```python
from build123d import *

# Parameters (mm, degrees)
BOSS_EXTRUDE1_START     = -5
BOSS_EXTRUDE1_OUTLINE_W = 200
BOSS_EXTRUDE1_OUTLINE_H = 70
BOSS_EXTRUDE1_OUTLINE_R = 2.25
BOSS_EXTRUDE1_DEPTH     = 5
BOSS_EXTRUDE2_START     = 3
SKETCH2_W               = 200
SKETCH2_H               = 65
SKETCH2_R               = 2.25
BOSS_EXTRUDE2_DEPTH     = 3
CHAMFER1_SIZE           = 8
CHAMFER3_SIZE           = 3
SKETCH3_W               = 7.071067812
SKETCH3_H               = 2.6
CUT_EXTRUDE1_DEPTH      = 224.573349607


# Read off the part's stored shape, not the designer's step: Boss-Extrude1
with BuildPart() as part:
    # Boss-Extrude1 outline → Boss-Extrude1 (new body)
    with BuildSketch(Plane.XY.offset(BOSS_EXTRUDE1_START)):
        with Locations((100, 35)):
            Rectangle(BOSS_EXTRUDE1_OUTLINE_W, BOSS_EXTRUDE1_OUTLINE_H)
        with Locations((20, 9)):
            Circle(BOSS_EXTRUDE1_OUTLINE_R, mode=Mode.SUBTRACT)
        with Locations((180, 9)):
            Circle(BOSS_EXTRUDE1_OUTLINE_R, mode=Mode.SUBTRACT)
        with Locations((20, 58)):
            Circle(BOSS_EXTRUDE1_OUTLINE_R, mode=Mode.SUBTRACT)
        with Locations((180, 58)):
            Circle(BOSS_EXTRUDE1_OUTLINE_R, mode=Mode.SUBTRACT)
    extrude(amount=BOSS_EXTRUDE1_DEPTH)

    # Sketch2 → Boss-Extrude2 (add)
    with BuildSketch(Plane(origin=(0, 0, -5), x_dir=(-1, 0, 0), z_dir=(0, 0, -1)).offset(BOSS_EXTRUDE2_START)):
        with Locations((-100, 37.5)):
            Rectangle(SKETCH2_W, SKETCH2_H)
        with Locations(Location((-20, 9, 0), (0, 0, 180))):
            Circle(SKETCH2_R, mode=Mode.SUBTRACT)
        with Locations((-180, 9)):
            Circle(SKETCH2_R, mode=Mode.SUBTRACT)
        with Locations(Location((-20, 58, 0), (0, 0, 180))):
            Circle(SKETCH2_R, mode=Mode.SUBTRACT)
        with Locations((-180, 58)):
            Circle(SKETCH2_R, mode=Mode.SUBTRACT)
    extrude(amount=-BOSS_EXTRUDE2_DEPTH)

    # Chamfer1
    # the kernel refuses this chamfer: 8 mm, written as the material it takes off along each edge
    with BuildSketch(Plane(origin=(200, -15.573463904, -8), x_dir=(-0.9996219169112968, 0, -0.027495876610586296), z_dir=(0, 1, 0)), Plane(origin=(0, 90.573463904, -8), x_dir=(0.9996219169112968, 0, -0.027495876610586275), z_dir=(0, -1, 0))) as chamfer1_piece_1:
        Polygon((CHAMFER1_SIZE * 0.999621916911, CHAMFER1_SIZE * 0.0274958766106), (-CHAMFER1_SIZE * 0.0274958766106, CHAMFER1_SIZE * 0.999621916911), (0, 0), align=None)
    extrude(amount=106.146927807, mode=Mode.SUBTRACT)

    # Chamfer3
    chamfer3_edges = [part.edges().sort_by_distance(p)[0] for p in [
        (100, 70, -8),
    ]]
    chamfer(chamfer3_edges, length=CHAMFER3_SIZE)

    # Sketch3 → Cut-Extrude1 (cut, through all, along a direction that is not the sketch's normal)
    with BuildSketch(Plane(origin=(100, 0, -100), x_dir=(-0.7071067811865452, 0, -0.7071067811865498), z_dir=(0.7071067811865498, 0, -0.7071067811865452))):
        with Locations((-137.885822331, 1.3)):
            Rectangle(SKETCH3_W, SKETCH3_H)
    extrude(amount=-CUT_EXTRUDE1_DEPTH, dir=(1, 0, 0), mode=Mode.SUBTRACT)


solid = part.part
```
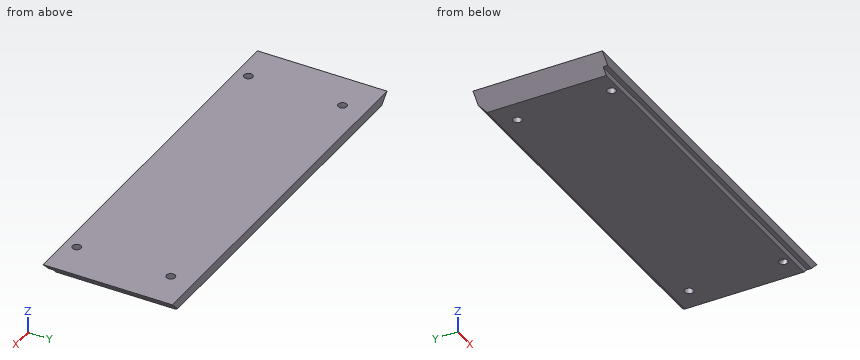
Can you work these out from the model? Positions are in its coordinate system, mm. Coordinates: 2 decimals unless noted, no trailing zeros. Loops run counter-clockwise (first coordinate to the right, second up) from the corner with the lowest first, then second, coordinate; pieces in that order, holes last. Notation, with made-up numbers: (28.25, 28) -> (58.25, 28) arc R12 cw to (58.25, 51) -> close; hole circle Ø11 at (79, 49). An arc over 180 degrees is marked (long way). Put each result on its own line as item: value. Start each with the question number.
Q1. I want a section at D-D (x = 142). Write out the boundary of the cut face in (y, z), plus the area to 4 significant figures.
Q2. I want a section at C-C (z = -2). Write out the boundary of the cut face in (x, y), plus the area to 3 significant figures.
Q3. I want a section at A-A (y = 58). Write out the boundary of the cut face in (x, z).
Q4. I'm going to push flat-ended pins straight in: P1, Ø4, axis at x = 20, y = 9, coming from the +Z side; P2, Ø4, axis at y = 31, z = -4, coming from the +X side; P3, Ø1.5, axis at x = 112.5, z = -6, coming from the -Y side; P4, Ø2, axis at y = 26, z = -5.5, coming from the -X side. Where does each tip first touch, or does it pass through?
Q5. If I drill on line 1 (Y direction, x = 180, z = -1.95); line 2 (X direction, y = 58, z = -5.6); line 3 (X direction, y = 58.5, z = -5.25), over which ranges is the centre line in solid material (lowest first)? Write a range as [from, to].
Taken from the geometry:
1. outline: (2.6, -5) -> (5, -5) -> (5, -8) -> (67, -8) -> (70, -5) -> (70, 0) -> (2.6, 0) -> close
1. area: 527.5 mm2
2. outline: (2, 2.6) -> (198, 2.6) -> (198, 70) -> (2, 70) -> close; hole circle Ø4.5 at (20, 9); hole circle Ø4.5 at (20, 58); hole circle Ø4.5 at (180, 9); hole circle Ø4.5 at (180, 58)
2. area: 13,100 mm2
3. outline: (0, 0) -> (8, -8) -> (17.75, -8) -> (17.75, 0) -> close; (22.25, -8) -> (177.75, -8) -> (177.75, 0) -> (22.25, 0) -> close; (182.25, -8) -> (192, -8) -> (200, 0) -> (182.25, 0) -> close
4. P1: passes through
4. P2: stops at x = 198
4. P3: stops at y = 5
4. P4: stops at x = 4.5
5. line 1: y = [2.6, 6.75], [11.25, 55.75], [60.25, 70]
5. line 2: x = [5.6, 17.75], [22.25, 177.75], [182.25, 194.4]
5. line 3: x = [5.25, 17.81], [22.19, 177.81], [182.19, 194.75]
